Work out the finished part from the listing and answer in its coordinate system (mm). Round coordinates to 2 decimals unless told otherwise and drop trailing zeros. Write each loop counter-clockwise with the first axis right and the second up, starting at its lowest first coordinate (ties: lowest second). Pieces come first, ordered by that corner, then holes. Notation, with made-up numbers: M 19,20 L 36,20 A22 cw 36,33 Z; hole C 32,-25.75 d5. An arc over 180 degrees is marked long. One line per item, written item: value. Start each with the question number.
Q1. Given pin 1 Ø8.5 at (x, y) = (46.99, 25.4) entering from +Z; pin 2 Ø1.5 at (y, z) = (-42.5, 1) entering from +X; pin 3 Ø2 at (x, z) = (-45.5, 0.5) entering from +Y; pin 4 Ø1.6 at (x, z) = (62, 3.5) entering from -Y, each flat-ended and moving along its own axis, determine where each tip first touches the part or whether it passes through.
Q2. Find section C-C (y = 49). Write down the section's boundary in (x, z), and give its area (3 significant figures).
Q3. Find section B-B (x = -8). Count the separate pieces of the cut face and the enclosed holes in it, and give its area (3 significant figures).
Q4. The mould has two halves that part along Y. Classify faces 1 (the cylindrical face through (-43.96, -24.45, 2.66)), 2 (the flat face through (-16, 1, 0)): released by +Y, released by -Y, zero draft, split by the parting line, or undercut.
Q5. Find section A-A (y = -18.5). Write down the section's boundary in (x, z), and give its area (3 significant figures).
Q6. Consider probe 1 along X at (y, z) = (17.5, 1); probe 2 along Y at (x, z) = (-19.5, 1.9); probe 3 along X at (y, z) = (44, 2.55). Determine where each line is inside the solid, lowest interval first.
from build123d import *

# Parameters (mm, degrees)
SKETCH1_R                = 1.651
BOSS_EXTRUDE2_DEPTH      = 5.3975
BOSS_EXTRUDE3_DEPTH      = 5.3975
FILLET1_R                = 1.27
SKETCH5_W                = 36.105919561
SKETCH5_H                = 30.801250688
SKETCH5_W_2              = 35.958513686
SKETCH5_H_2              = 33.469345806
BOSS_EXTRUDE4_DEPTH      = 5.3975
SKETCH7_R                = 3.175
CUT_EXTRUDE4_DEPTH       = 234.082045613
CUT_EXTRUDE4_DEPTH_BACK  = 234.082045613
SKETCH8_R                = 4.445
BOSS_EXTRUDE5_DEPTH      = 5.3975
SKETCH12_R               = 12.192
CUT_EXTRUDE8_DEPTH       = 154.925374637
CUT_EXTRUDE8_DEPTH_BACK  = 154.925374637
SKETCH14_R               = 12.192
CUT_EXTRUDE10_DEPTH      = 38.862
SKETCH15_R               = 3.937
CUT_EXTRUDE11_DEPTH      = 21.59
SKETCH16_R               = 1.651
CUT_EXTRUDE12_DEPTH      = 150.876
SKETCH17_R               = 3.175
CUT_EXTRUDE13_DEPTH      = 103.378
CUT_EXTRUDE13_DEPTH_BACK = 48.768


with BuildPart() as part:
    # Sketch1 → Boss-Extrude2 (new body)
    with BuildSketch(Plane.XY):
        with BuildLine():
            Line((-68.336857873, 30.734), (-55.636857873, 30.734))
            Line((-55.636857873, 30.734), (-55.636857873, -30.734))
            Line((-55.636857873, -30.734), (-68.336857873, -30.734))
            ThreePointArc((-68.336857873, -30.734), (0, -74.93), (68.336857873, -30.734))
            Line((68.336857873, -30.734), (55.636857873, -30.734))
            Line((55.636857873, -30.734), (55.636857873, 30.734))
            Line((55.636857873, 30.734), (68.336857873, 30.734))
            ThreePointArc((68.336857873, 30.734), (0, 74.93), (-68.336857873, 30.734))
        make_face()
        with Locations((-45.466, 11.049)):
            Circle(SKETCH1_R, mode=Mode.SUBTRACT)
        with Locations((-20.067270032, 10.795)):
            Circle(SKETCH1_R, mode=Mode.SUBTRACT)
        with Locations(Location((-20.067270032, -10.795, 0), (0, 0, 180))):
            Circle(SKETCH1_R, mode=Mode.SUBTRACT)
        with Locations(Location((-45.466, -11.049, 0), (0, 0, 180))):
            Circle(SKETCH1_R, mode=Mode.SUBTRACT)
        with Locations((45.466, -11.049)):
            Circle(SKETCH1_R, mode=Mode.SUBTRACT)
        with Locations((20.067270032, -10.795)):
            Circle(SKETCH1_R, mode=Mode.SUBTRACT)
        with Locations(Location((20.067270032, 10.795, 0), (0, 0, 180))):
            Circle(SKETCH1_R, mode=Mode.SUBTRACT)
        with Locations(Location((45.466, 11.049, 0), (0, 0, 180))):
            Circle(SKETCH1_R, mode=Mode.SUBTRACT)
    extrude(amount=BOSS_EXTRUDE2_DEPTH)

    # Sketch4 → Boss-Extrude3 (add)
    with BuildSketch(Plane(origin=(0, 0, 0), x_dir=(-1, 0, 0), z_dir=(0, 0, -1))):
        with BuildLine():
            Line((-68.336857873, -30.734), (-67.320857873, -30.734))
            Line((-67.320857873, -30.734), (-67.320857873, 30.734))
            Line((-67.320857873, 30.734), (-68.336857873, 30.734))
            ThreePointArc((-68.336857873, 30.734), (-74.93, 0), (-68.336857873, -30.734))
        make_face()
        with BuildLine():
            Line((67.320857873, 30.734), (68.336857873, 30.734))
            ThreePointArc((68.336857873, 30.734), (74.93, 0), (68.336857873, -30.734))
            Line((68.336857873, -30.734), (67.320857873, -30.734))
            Line((67.320857873, -30.734), (67.320857873, 30.734))
        make_face()
    extrude(amount=-BOSS_EXTRUDE3_DEPTH)

    # Fillet1
    fillet1_edges = [part.edges().sort_by_distance(p)[0] for p in [
        (67.320857873, -30.734, 2.69875),
        (67.320857873, 30.734, 2.69875),
        (-67.320857873, 30.734, 2.69875),
        (-67.320857873, -30.734, 2.69875),
    ]]
    fillet(fillet1_edges, radius=FILLET1_R)

    # Sketch5 → Boss-Extrude4 (add)
    with BuildSketch(Plane(origin=(0, 0, 0), x_dir=(-1, 0, 0), z_dir=(0, 0, -1))):
        with Locations((34.78484389, -0.38515144)):
            Rectangle(SKETCH5_W, SKETCH5_H)
        with Locations((-32.830563904, 0.948896119)):
            Rectangle(SKETCH5_W_2, SKETCH5_H_2)
    extrude(amount=-BOSS_EXTRUDE4_DEPTH)

    # Sketch7 → Cut-Extrude4 (cut, two sides)
    with BuildSketch(Plane(origin=(30.087765895, -133.08292226, 0), x_dir=(-0.008405041193852665, -0.9999646770174084, 0), z_dir=(0, 0, 1))) as cut_extrude4_sk:
        with Locations(Location((-157.958959999, 14.406563609, 0), (0, 0, 90.481579057))):
            Circle(SKETCH7_R)
        with Locations(Location((-173.198959999, -31.313436391, 0), (0, 0, 90.481579057))):
            Circle(SKETCH7_R)
        with Locations(Location((-157.958959999, -77.033436391, 0), (0, 0, 270.481579057))):
            Circle(SKETCH7_R)
        with Locations(Location((-107.158959999, -77.033436391, 0), (0, 0, 90.481579057))):
            Circle(SKETCH7_R)
        with Locations(Location((-91.918959999, -31.313436391, 0), (0, 0, 270.481579057))):
            Circle(SKETCH7_R)
        with Locations(Location((-107.158959999, 14.406563609, 0), (0, 0, 270.481579057))):
            Circle(SKETCH7_R)
    extrude(amount=CUT_EXTRUDE4_DEPTH, mode=Mode.SUBTRACT)
    extrude(cut_extrude4_sk.sketch, amount=-CUT_EXTRUDE4_DEPTH_BACK, mode=Mode.SUBTRACT)

    # Sketch8 → Boss-Extrude5 (add)
    with BuildSketch(Plane(origin=(0, 0, 0), x_dir=(-1, 0, 0), z_dir=(0, 0, -1))):
        with Locations((-45.821472187, 24.749370396)):
            Circle(SKETCH8_R)
        with Locations((-0.231179981, 40.373110558)):
            Circle(SKETCH8_R)
        with Locations((45.61529788, 25.517927363)):
            Circle(SKETCH8_R)
        with Locations((46.042273972, -25.280278229)):
            Circle(SKETCH8_R)
        with Locations((0.451981767, -40.90401839)):
            Circle(SKETCH8_R)
        with Locations((-45.394496094, -26.048835196)):
            Circle(SKETCH8_R)
    extrude(amount=-BOSS_EXTRUDE5_DEPTH)

    # Sketch12 → Cut-Extrude8 (cut, two sides)
    with BuildSketch(Plane(origin=(54.141453623, -7.598175858, -9.525), x_dir=(-1, 0, 0), z_dir=(0, 0, -1))) as cut_extrude8_sk:
        with Locations((11.215453623, 50.524175858)):
            Circle(SKETCH12_R)
        with Locations((38.363844634, 66.481014229)):
            Circle(SKETCH12_R)
        with Locations((39.917453623, 41.888175858)):
            Circle(SKETCH12_R)
        with Locations((54.141453623, 7.598175858)):
            Circle(SKETCH12_R)
        with Locations(Location((69.919062613, 66.481014229, 0), (0, 0, 180))):
            Circle(SKETCH12_R)
        with Locations(Location((68.365453623, 41.888175858, 0), (0, 0, 180))):
            Circle(SKETCH12_R)
        with Locations(Location((97.067453623, 50.524175858, 0), (0, 0, 180))):
            Circle(SKETCH12_R)
        with Locations((68.365453623, -26.691824142)):
            Circle(SKETCH12_R)
        with Locations((97.067453623, -35.327824142)):
            Circle(SKETCH12_R)
        with Locations((69.919062613, -51.284662512)):
            Circle(SKETCH12_R)
        with Locations(Location((38.363844634, -51.284662512, 0), (0, 0, 180))):
            Circle(SKETCH12_R)
        with Locations(Location((11.215453623, -35.327824142, 0), (0, 0, 180))):
            Circle(SKETCH12_R)
        with Locations(Location((39.917453623, -26.691824142, 0), (0, 0, 180))):
            Circle(SKETCH12_R)
    extrude(amount=CUT_EXTRUDE8_DEPTH, mode=Mode.SUBTRACT)
    extrude(cut_extrude8_sk.sketch, amount=-CUT_EXTRUDE8_DEPTH_BACK, mode=Mode.SUBTRACT)

    # Sketch14 → Cut-Extrude10 (cut)
    with BuildSketch(Plane(origin=(0, 0, 0), x_dir=(-1, 0, 0), z_dir=(0, 0, -1))):
        with Locations((-31.75, 0)):
            Circle(SKETCH14_R)
        with Locations(Location((31.75, 0, 0), (0, 0, 180))):
            Circle(SKETCH14_R)
        with BuildLine():
            Line((-12.7, 20.32), (12.7, 20.32))
            ThreePointArc((12.7, 20.32), (19.05, 13.97), (12.7, 7.62))
            ThreePointArc((12.7, 7.62), (0, 13.754080301), (-12.7, 7.62))
            ThreePointArc((-12.7, 7.62), (-19.05, 13.97), (-12.7, 20.32))
        make_face()
        with BuildLine():
            Line((-12.7, -20.32), (12.7, -20.32))
            ThreePointArc((12.7, -20.32), (19.05, -13.97), (12.7, -7.62))
            ThreePointArc((12.7, -7.62), (0, -13.754080301), (-12.7, -7.62))
            ThreePointArc((-12.7, -7.62), (-19.05, -13.97), (-12.7, -20.32))
        make_face()
    extrude(amount=-CUT_EXTRUDE10_DEPTH, mode=Mode.SUBTRACT)

    # Sketch15 → Cut-Extrude11 (cut)
    with BuildSketch(Plane(origin=(0, 0, 0), x_dir=(-1, 0, 0), z_dir=(0, 0, -1))):
        with Locations((0, -66.04)):
            Circle(SKETCH15_R)
        with Locations(Location((0, 66.04, 0), (0, 0, 180))):
            Circle(SKETCH15_R)
    extrude(amount=-CUT_EXTRUDE11_DEPTH, mode=Mode.SUBTRACT)

    # Sketch16 → Cut-Extrude12 (cut)
    with BuildSketch(Plane(origin=(-30.092005081, 4.08352975, -57.7215), x_dir=(-1, 0, 0), z_dir=(0, 0, -1))):
        with Locations(Location((-101.395980802, -12.71952975, 0), (0, 0, 180))):
            Circle(SKETCH16_R)
        with Locations(Location((-101.395980802, 4.55247025, 0), (0, 0, 180))):
            Circle(SKETCH16_R)
        with Locations(Location((41.211970641, -12.71952975, 0), (0, 0, 180))):
            Circle(SKETCH16_R)
        with Locations(Location((41.211970641, 4.55247025, 0), (0, 0, 180))):
            Circle(SKETCH16_R)
    extrude(amount=-CUT_EXTRUDE12_DEPTH, mode=Mode.SUBTRACT)

    # Sketch17 → Cut-Extrude13 (cut, two sides)
    with BuildSketch(Plane(origin=(-30.092005081, 4.08352975, -46.9265), x_dir=(1, 0, 0), z_dir=(0, 0, 1))) as cut_extrude13_sk:
        with Locations((-16.897994919, 21.31647025)):
            Circle(SKETCH17_R)
        with Locations((77.082005081, 21.31647025)):
            Circle(SKETCH17_R)
        with Locations((30.092005081, 21.31647025)):
            Circle(SKETCH17_R)
        with Locations((77.082005081, -29.48352975)):
            Circle(SKETCH17_R)
        with Locations((30.092005081, -29.48352975)):
            Circle(SKETCH17_R)
        with Locations((-16.897994919, -29.48352975)):
            Circle(SKETCH17_R)
    extrude(amount=CUT_EXTRUDE13_DEPTH, mode=Mode.SUBTRACT)
    extrude(cut_extrude13_sk.sketch, amount=-CUT_EXTRUDE13_DEPTH_BACK, mode=Mode.SUBTRACT)


solid = part.part
The answers:
1. pin 1: z = 5.4
1. pin 2: x = 62.22
1. pin 3: y = 60.28
1. pin 4: y = -43.23
2. outline: M -56.69,0 L -53.5,0 L -53.5,5.4 L -56.69,5.4 Z; M -32.35,0 L -22.92,0 L -22.92,5.4 L -32.35,5.4 Z; M -8.64,0 L 8.64,0 L 8.64,5.4 L -8.64,5.4 Z; M 22.92,0 L 32.35,0 L 32.35,5.4 L 22.92,5.4 Z; M 53.5,0 L 56.69,0 L 56.69,5.4 L 53.5,5.4 Z
2. area: 230 mm2
3. separate pieces: 8
3. enclosed holes: 0
3. area: 182 mm2
4. face 1: undercut
4. face 2: zero draft
5. outline: M -72.61,0 L -67.32,0 L -67.32,5.4 L -72.61,5.4 Z; M -55.64,0 L -17.15,0 L -17.15,5.4 L -55.64,5.4 Z; M 17.15,0 L 55.64,0 L 55.64,5.4 L 17.15,5.4 Z; M 67.32,0 L 72.61,0 L 72.61,5.4 L 67.32,5.4 Z
5. area: 473 mm2
6. probe 1: -72.86 to -67.32, -55.64 to -17.98, 17.98 to 55.64, 67.32 to 72.86
6. probe 2: -72.35 to -70.49, -47.27 to -45.28, -23.3 to 23.3, 45.28 to 47.27, 70.49 to 72.35
6. probe 3: -60.65 to -55.07, -30.78 to -21.6, -6.85 to 6.85, 21.6 to 30.78, 55.07 to 60.65
